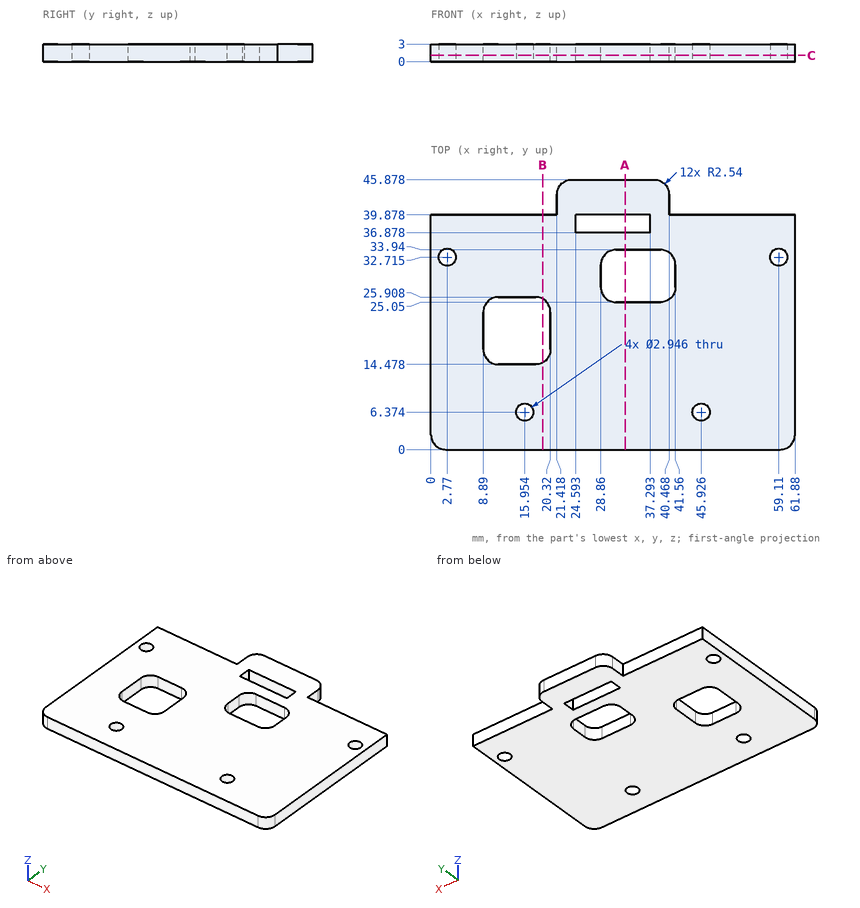
Answer from the drawing. Dimensions are ordinates in mm from the lowest x, y and z of the part. Round coordinates to 2 decimals unless told otherwise and drop trailing zeros. Loops run counter-clockwise (first coordinate to the right, second up) from the corner with the lowest first, then second, coordinate; pieces in that order, holes last.
(1) The part is cut by section A-A, the plane x = 33. Give the vertices of the cut face in (y, z).
Computed values:
outline: (0, 0) - (25.05, 0) - (25.05, 3) - (0, 3) - close; (33.94, 0) - (36.88, 0) - (36.88, 3) - (33.94, 3) - close; (39.88, 0) - (45.88, 0) - (45.88, 3) - (39.88, 3) - close
(2) This flat-tipped pin is pushed along its axis until it touches: P1, Ø1.5, axis at x = 13.5, z = 2, coming from the +Y side. Where does it stop, or does it pass through?
Computed values:
P1: stops at y = 39.88
(3) The part is cut by section C-C, the plane z = 1.05. Give the number of separate pieces and of enclosed holes in the cut face, and give its area (3 significant figures).
Computed values:
separate pieces: 1
enclosed holes: 7
area: 2,280 mm2
(4) The part is cut by section B-B, the plane x = 19. Give the vertices of the cut face in (y, z).
Computed values:
outline: (0, 0) - (14.79, 0) - (14.79, 3) - (0, 3) - close; (25.6, 0) - (39.88, 0) - (39.88, 3) - (25.6, 3) - close
(5) Find the intervals of material crossed by L1, parallel to Y at x = 16, z = 0.2; L2, parallel to X at y = 29, z = 2.4; L3, parallel to Y at x = 59.11, z = 1.85, in increasing order.
Computed values:
L1: y = 0 to 4.9, 7.85 to 14.48, 25.91 to 39.88
L2: x = 0 to 28.86, 41.56 to 61.88
L3: y = 0 to 31.24, 34.19 to 39.88
